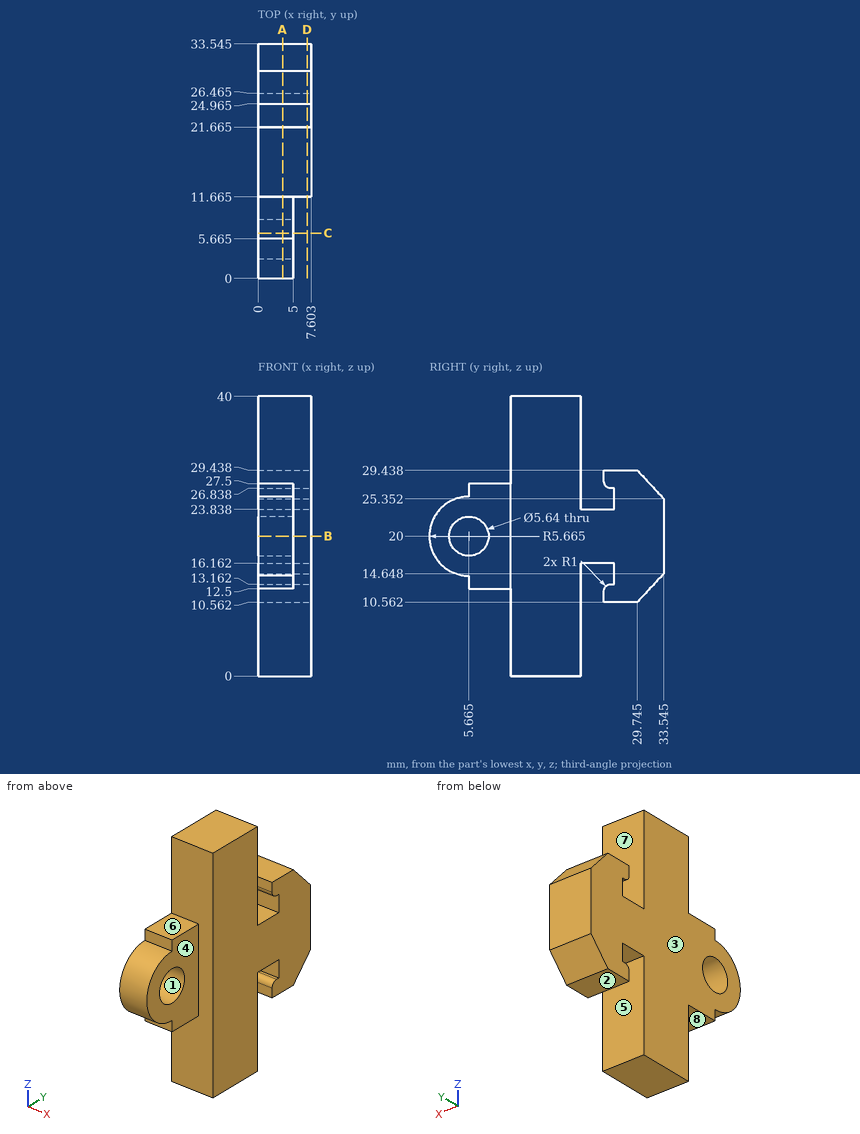
Geometry check sheet. Reference: drawing and pictorial views, mm from the part's lowest x, y, z. A direction names the side the tool comes from. Give positions to 0.01 mm unless a question says otherwise; leave off trailing zeros. Write each loop counter-clockwise with the first axis right and the second up, starting at its lowest first coordinate (ties: lowest second). Pieces come first, ordered by that corner, then holes. Notation, with made-up numbers: M -33.5,11.5 L 2.5,11.5 A20 ccw 2.5,24.5 Z; hole C -11,66.5 d9. An arc over 180 degrees is marked long. Answer as CSV lines item,"result". Start each with the question number.
Q1. Section check A-A, the plane x = 3.5. Record the cut outline in (y, z) (1 decimal), then the cut area to 3 significant figures.
Q2. Section check D-D, the plane x = 7. Record the cut outline in (y, z) (1 decimal).
Q3. Material ranges on L1, parallel to Y at x = 1.95, z = 20 (1 decimal); L2, parallel to Y at x = 4.5, z = 32 (1 decimal); L3, parallel to Z at x = 1, y = 22.5, recorded low to high.
Q4. Section check C-C, the plane y = 6.5. Record the cut outline in (x, z).
Q5. Tool access check on the marked faces 4, 5, 6, 7 and 8. Record the directions out of +Z, -Z, +X, -X, +Y, -Y that give a thin tool (end or side, any length) a straight path to the whole face; none if there is none.
Q6. Section check B-B, the plane z = 20. Record the cut outline in (x, y) (1 decimal).
Q7. Release check for a two-part mould opening along Z. For the marked faces 1, 2 and 3 record: pulls with the +Z half, pulls with the -Z half, needs draft (parallel to the pull), parting line crosses it, or undercut.
Q8. Go/stop test with flat-tipped pins: pin 1 (7.5 mm diameter, centred on y = 5.665, z = 20, fed in from +X); pin 2 (1.5 mm diameter, centred on x = 2, z = 14, fed in from -Y) (1 decimal); pin 3 (4 mm diameter, centred on x = 3, y = 9.5, fed in from -Z). Record where each tip stops, or that it passes through.
Geometry says:
1,outline,"M 5.7,12.5 L 11.7,12.5 L 11.7,0 L 21.7,0 L 21.7,16.2 L 26.5,16.2 L 26.5,13.2 L 26,13.2 A1 ccw 25,12.2 L 25,10.6 L 29.7,10.6 L 33.5,14.6 L 33.5,25.4 L 29.7,29.4 L 25,29.4 L 25,27.8 A1 ccw 26,26.8 L 26.5,26.8 L 26.5,23.8 L 21.7,23.8 L 21.7,40 L 11.7,40 L 11.7,27.5 L 5.7,27.5 L 5.7,25.7 A5.7 ccw 5.7,14.3 Z; hole C 5.7,20 d5.6"
1,area,"678 mm^2"
2,outline,"M 11.7,0 L 21.7,0 L 21.7,16.2 L 26.5,16.2 L 26.5,13.2 L 26,13.2 A1 ccw 25,12.2 L 25,10.6 L 29.7,10.6 L 33.5,14.6 L 33.5,25.4 L 29.7,29.4 L 25,29.4 L 25,27.8 A1 ccw 26,26.8 L 26.5,26.8 L 26.5,23.8 L 21.7,23.8 L 21.7,40 L 11.7,40 Z"
3,L1,"0 to 2.8, 8.5 to 33.5"
3,L2,"11.7 to 21.7"
3,L3,"16.16 to 23.84"
4,outline,"M 0,12.5 L 5,12.5 L 5,17.31 L 0,17.31 Z; M 0,22.69 L 5,22.69 L 5,27.5 L 0,27.5 Z"
5,face 4,"+Z, -Z, +X, -Y"
5,face 5,"-Z, +X, -X"
5,face 6,"+Z, +X, -X, -Y"
5,face 7,"+Z, +X, -X"
5,face 8,"-Z, +X, -X, -Y"
6,outline,"M 0,0 L 5,0 L 5,2.8 L 0,2.8 Z; M 0,8.5 L 5,8.5 L 5,11.7 L 7.6,11.7 L 7.6,33.5 L 0,33.5 Z"
7,face 1,"undercut"
7,face 2,"pulls with the -Z half"
7,face 3,"needs draft"
8,pin 1,"x = 5"
8,pin 2,"y = 3.5"
8,pin 3,"z = 12.5"
